from build123d import *

# Parameters (mm, degrees)
F0_R     = 53
F0_R_2   = 50
F1_DEPTH = 300
F3_DEPTH = 300.001
F4_R     = 15
F5_R     = 1


with BuildPart() as f1:
    # F0 (on Right) → F1 (new body)
    with BuildSketch(Plane.YZ):
        with Locations((0, 1.8706418186)):
            Circle(F0_R)
        with Locations((0, 1.8706418186)):
            Circle(F0_R_2, mode=Mode.SUBTRACT)
    extrude(amount=F1_DEPTH)

    # F2 (on Right) → F3 (cut, through all)
    with BuildSketch(Plane.YZ):
        Polygon((-45, 0), (0, 0), (150.288850058, 0), (150.288850058, 138.1199563971), (0, 138.1199563971), (-236.3291914778, 138.1199563971), (-236.3291914778, 0), (-65, 0), (-65, 5), (-45, 5), align=None)
    extrude(amount=F3_DEPTH, mode=Mode.SUBTRACT)

    # F4
    f4_edges = [f1.edges().sort_by_distance(p)[0] for p in [
        (300, 51.465986, 0),
        (0, 51.465986, 0),
    ]]
    fillet(f4_edges, radius=F4_R)

    # F5
    f5_edges = [f1.edges().sort_by_distance(p)[0] for p in [
        (150, 52.966977, 0),
        (285, 51.465986, 0),
        (15, 51.465986, 0),
        (150, 49.964995, 0),
    ]]
    fillet(f5_edges, radius=F5_R)


solid = f1.part
Here's how the part is built. I have some questions about the finished solid (model axes, mm). A direction names the side the tool comes from. Round coordinates to 2 decimals unless told otherwise and drop trailing zeros. Order: outer loops, then holes, each group sorted by start corner. A loop starts at its lowest first (then second) coordinate and runs counter-clockwise, first axis right, second up. Notation, with made-up numbers: (-22.5, 54) -> (-7.5, 54) arc R28 ccw to (-7.5, 77) -> close; hole circle Ø2 at (13, -11.75). An arc over 180 degrees is marked (long way). Return JSON: item names as keys, results as strings.
Q1. I need wall thicknesses on line 1 along Y through (x, z) = (251, -31); line 2 along Y through (x, z) = (258, -7); line 3 along Z through (x, y) = (46.5, -32.5). Which ranges of each line are inside material? Lowest first, please. Write a range as from..to.
Filled sheet:
{"line 1": "y = -41.58..-37.68, 37.68..41.58", "line 2": "y = -52.25..-49.21, 49.21..52.25", "line 3": "z = -40..-36.13"}
Q2. If we section it at A-A on y = 0: List the corners of the cut face in (x, z) for me.
Filled sheet:
{"outline": "(0, -50.13) arc R1 ccw to (1, -51.13) -> (299, -51.13) arc R1 ccw to (300, -50.13) -> (300, -49.13) arc R1 ccw to (299, -48.13) -> (1, -48.13) arc R1 ccw to (0, -49.13) -> close"}
Q3. For pin 1 Ø5 at (x, y) = (126.5, 14.5) entering from -Z; pin 2 Ø10 at (x, z) = (115.5, -7) entering from +Y; pin 3 Ø5 at (x, z) = (89.5, -4) entering from -Y; pin 4 Ø6 at (y, z) = (-14, -40.5) entering from +X, each with a flat end and sliding along its axis, tell me the tip position at first contact or that it passes through.
Filled sheet:
{"pin 1": "stops at z = -49.75", "pin 2": "stops at y = 52.86", "pin 3": "stops at y = -52.89", "pin 4": "passes through"}
Q4. If we mould it in two halves opening along Y, with no side actions, what happens to faces 1 (the flat face through (300, 6, -49)), 2 (the cylindrical face through (147.914, -4.192, -50.963)), 3 (the cylindrical face through (147.914, -4.071, -47.963))? For each: released by +Y, released by -Y, zero draft, split by the parting line, or undercut.
Filled sheet:
{"face 1": "zero draft", "face 2": "split by the parting line", "face 3": "undercut"}
Q5. Which directions (+Z, -Z, +X, -X, +Y, -Y) give clear straight access to the entire face, cutting with the end or side of a thin tool? Please do faces 4 (the flat face through (0, 6, -49)), 5 (the cylindrical face through (4.355, 50.736, -4.432)), 6 (the cylindrical face through (295.568, 50.859, -4.355)).
Filled sheet:
{"face 4": "+Z, -Z, -X, +Y, -Y", "face 5": "+Z, -X, +Y", "face 6": "+Z, +X, +Y"}
